The model under review builds one solid part; all positions refer to its coordinate system, in mm. Round coordinates to 2 decimals unless told otherwise and drop trailing zeros. Loops run counter-clockwise (first coordinate to the right, second up) from the corner with the lowest first, then second, coordinate; pieces in that order, holes last. Notation, with made-up numbers: M -35,14 L 12,14 A18 ccw 12,27 Z; hole C 16,37.5 d1. An arc over 180 degrees is marked long. Use a Markdown table: item, result. Add a question column.
```python
from build123d import *

# Parameters (mm, degrees)
F2_R     = 19.05
F3_DEPTH = 25.4
F4_DEPTH = 127
F5_SIZE  = 19.05


with BuildPart() as f1:
    # F0 (on Front) → F1 (revolve)
    with BuildSketch(Plane.XZ):
        with BuildLine():
            Line((0, 0), (0, 53.77469))
            ThreePointArc((0, 53.77469), (-53.77469, 0), (0, -53.77469))
            Line((0, -53.77469), (0, 0))
        make_face()
    revolve(axis=Axis((0, 0, 26.887345), (0, 0, -1)))



with BuildPart() as f3:
    # F2 (on Top) → F3 (new body)
    with BuildSketch(Plane.XY):
        Circle(F2_R)
    extrude(amount=-F3_DEPTH)


with BuildPart() as f1_1:
    add(f1.part)

    add(f3.part)  # F4 merges F3
    # F2 (on Top) → F4 (join)
    with BuildSketch(Plane.XY):
        Circle(F2_R)
    extrude(amount=F4_DEPTH)

    # F5
    f5_edges = [f1_1.edges().sort_by_distance(p)[0] for p in [
        (-19.05, 0, 127),
    ]]
    chamfer(f5_edges, length=F5_SIZE)


solid = f1_1.part
```
(1) Insertion check: pin 1 Ø12 at (x, z) = (-41.5, -33) entering from +Y; pin 2 Ø5 at (x, y) = (6.5, 41.5) entering from +Z; pin 3 Ø1 at (x, y) = (2, 31.5) entering from -Z. Each pin has a flat end and moves straight along its axis. Give the tip position at first contact, or say it passes through.
(2) To check wall thickness, follow probe 1 along Y at (x, z) = (-46, 15); probe 2 along Y at (x, z) = (-18.5, -34); probe 3 along X at (y, z) = (7, -20.5). State the ranges of each line that lie inside material, in increasing order.
(3) Consider section B-B, the plane x = 24.5. Give the boundary of the cut face in (y, z), then the cut area to 3 significant figures.
(4) Consider section A-A, the plane z = 67. Give the boundary of the cut face in (x, y).
Found:
| question | item | result |
|---|---|---|
| 1 | pin 1 | stops at y = 26.09 |
| 1 | pin 2 | stops at z = 36.48 |
| 1 | pin 3 | stops at z = -43.9 |
| 2 | probe 1 | y = -23.47 to 23.47 |
| 2 | probe 2 | y = -37.33 to 37.33 |
| 2 | probe 3 | x = -49.22 to 49.22 |
| 3 | outline | C 0,0 d95.74 |
| 3 | area | 7,200 mm^2 |
| 4 | outline | C 0,0 d38.1 |
